```python
from build123d import *

# Parameters (mm, degrees)
SKETCH_1_W          = 165
SKETCH_1_H          = 31.5
EXTRUDE_1_DEPTH     = 29.6
SKETCH_2_R          = 12
SKETCH_2_R_2        = 10
SKETCH_2_R_3        = 5.5
SKETCH_2_R_4        = 4.5
CUT_EXTRUDE_1_DEPTH = 0.6
FILLET_1_R          = 4
FILLET_2_R          = 1
SKETCH_3_W          = 8
SKETCH_3_H          = 10
CUT_EXTRUDE_2_DEPTH = 4
CUT_EXTRUDE_3_DEPTH = 10
SCALE_1_SCALE       = 0.5


with BuildPart() as part:
    # 草图1 → 凸台-拉伸1 (new body)
    with BuildSketch(Plane.XY):
        Rectangle(SKETCH_1_W, SKETCH_1_H)
    extrude(amount=EXTRUDE_1_DEPTH)

    # 草图2 → 切除-拉伸1 (cut)
    # profile 1 of 4: a face of its own
    with BuildSketch(Plane.XY.offset(29.6)):
        with Locations((-60, 0)):
            Circle(SKETCH_2_R)
        with Locations((-60, 0)):
            Circle(SKETCH_2_R_2, mode=Mode.SUBTRACT)
    # profile 2 of 4: a face of its own
    with BuildSketch(Plane.XY.offset(29.6)):
        with Locations((-60, 0)):
            Circle(SKETCH_2_R_3)
        with Locations((-60, 0)):
            Circle(SKETCH_2_R_4, mode=Mode.SUBTRACT)
    # profile 3 of 4: a face of its own
    with BuildSketch(Plane.XY.offset(29.6)):
        with Locations((60, 0)):
            Circle(SKETCH_2_R)
        with Locations((60, 0)):
            Circle(SKETCH_2_R_2, mode=Mode.SUBTRACT)
    # profile 4 of 4: a face of its own
    with BuildSketch(Plane.XY.offset(29.6)):
        with Locations((60, 0)):
            Circle(SKETCH_2_R_3)
        with Locations((60, 0)):
            Circle(SKETCH_2_R_4, mode=Mode.SUBTRACT)
    extrude(amount=-CUT_EXTRUDE_1_DEPTH, mode=Mode.SUBTRACT)

    # 圆角1
    fillet_1_edges = [part.edges().sort_by_distance(p)[0] for p in [
        (82.5, -15.75, 14.8),
        (-82.5, -15.75, 14.8),
        (-82.5, 15.75, 14.8),
        (82.5, 15.75, 14.8),
    ]]
    fillet(fillet_1_edges, radius=FILLET_1_R)

    # 圆角2
    fillet_2_edges = [part.edges().sort_by_distance(p)[0] for p in [
        (82.5, 0, 0),
        (82.5, 0, 29.6),
        (0, -15.75, 0),
        (-82.5, 0, 0),
        (0, 15.75, 0),
        (-81.328427125, 14.578427125, 0),
        (-81.328427125, -14.578427125, 0),
        (81.328427125, 14.578427125, 0),
        (81.328427125, -14.578427125, 0),
        (0, -15.75, 29.6),
        (0, 15.75, 29.6),
        (-82.5, 0, 29.6),
        (-81.328427125, 14.578427125, 29.6),
        (-81.328427125, -14.578427125, 29.6),
        (81.328427125, 14.578427125, 29.6),
        (81.328427125, -14.578427125, 29.6),
    ]]
    fillet(fillet_2_edges, radius=FILLET_2_R)

    # 草图3 → 切除-拉伸2 (cut)
    with BuildSketch(Plane.XY.offset(29.6)):
        with Locations((-22, 0)):
            Rectangle(SKETCH_3_W, SKETCH_3_H)
        with Locations((22, 0)):
            Rectangle(SKETCH_3_W, SKETCH_3_H)
    extrude(amount=-CUT_EXTRUDE_2_DEPTH, mode=Mode.SUBTRACT)

    # 草图4 → 切除-拉伸3 (cut)
    with BuildSketch(Plane.XZ.offset(-5)):
        Polygon((26, 25.6), (44.574175621, 29.6), (26, 29.6), align=None)
        Polygon((-26, 29.6), (-44.574175621, 29.6), (-26, 25.6), align=None)
    extrude(amount=CUT_EXTRUDE_3_DEPTH, mode=Mode.SUBTRACT)


with BuildPart() as part_1:
    # 缩放比例1: scaled about (0, 0, 14.660574606)
    add(part.part.scale(SCALE_1_SCALE).moved(Location((0, 0, 7.330287303))))


solid = part_1.part
```
For this review, take the finished solid that the model builds, in its own axes (mm). A direction names the side the tool comes from. Coordinates: 2 decimals unless noted, no trailing zeros. Return JSON: item names as keys, results as strings. Group by question number.
(1) Mouldability with a two-part tool opening along Y and no side actions: class faces 1 (the cylindrical face through (-40.68, -7.274, 14.827)), 2 (the flat face through (-17.709, 0.035, 21.144)), 3 (the flat face through (-27.8, -2.2, 22.13)) as pulls with the +Y half, pulls with the -Y half, needs draft (parallel to the pull), parting line crosses it, or undercut.
(2) To check wall thickness, follow L1, parallel to Y at x = 30, z = 22; L2, parallel to Y at x = 30, z = 21.9; L3, parallel to Z at x = -9.5, y = 0.25. State the ranges of each line that lie inside material, in increasing order.
(3) Tool access review of faces 4 (the flat face through (30, 0, 22.13)), 5 (the flat face through (-14, -2.5, 21)): name each direction out of +Z, -Z, +X, -X, +Y, -Y from which nothing blocks a thin tool from reaching the whole face with its end or side.
(4) For pin 1 Ø1.2 at (x, y) = (11.5, -1) entering from +Z, flat-tipped, find the tip position at first contact; note if it passes through.
Results below:
{
 "1": {"face 1": "pulls with the -Y half", "face 2": "undercut", "face 3": "needs draft"},
 "2": {"L1": "y = -7.71 to -6, -5 to -2.75, -2.25 to 2.25, 2.75 to 5, 6 to 7.71", "L2": "y = -7.8 to -6, -5 to -2.75, -2.25 to 2.25, 2.75 to 5, 6 to 7.8", "L3": "z = 7.33 to 20.13"},
 "3": {"face 4": "+Z, +X, -X, +Y, -Y", "face 5": "+Z"},
 "4": {"pin 1": "stops at z = 20.13"}
}
